Geometry: final body of the model. Coordinates: model frame, mm. Round coordinates to 2 decimals unless told otherwise and drop trailing zeros. Order: outer loops, then holes, each group sorted by start corner. A loop starts at its lowest first (then second) coordinate and runs counter-clockwise, first axis right, second up. Notation, with made-up numbers: M 44,-39 L 73,-39 A17 ccw 73,-17 Z; hole C 36,81 d6. An arc over 180 degrees is marked long. Return JSON: item names as keys, results as strings. Group by question number.
Q1. Cut plane A-A on z = 1.7. Output: boundary loops of the cut face in (x, y).
Q2. Ray query, probe 1 along X at (y, z) = (20, 2.35); probe 2 along Y at (x, z) = (-14.6, 1.35); probe 3 along X at (y, z) = (32, 1.55). Return the intervals inside material, ascending.
Q3. Cut plane B-B on x = -410.5. Output: boundary loops of the cut face in (y, z) (3 decimals).
Q4. Contact query for flat-ended pins moving along their axis: pin 1 (1 mm diameter, centred on x = -445.5, z = 1, fed in from -Y); pin 2 (2 mm diameter, centred on x = -304, y = 116, fed in from -Z). Output: stop coordinate, or through.
Q5. Cut plane C-C on y = 30.5. Output: boundary loops of the cut face in (x, z) (3 decimals), and give its area (3 significant figures).
```python
from build123d import *

# Parameters (mm, degrees)
SKETCH1_R           = 3.05
BOSS_EXTRUDE1_DEPTH = 3.175


with BuildPart() as part:
    # Sketch1 → Boss-Extrude1 (new body)
    with BuildSketch(Plane.XY):
        with BuildLine():
            Line((-466, 88.2), (-466, 131.8))
            Line((-466, 131.8), (0, 131.8))
            Line((0, 131.8), (0, 0))
            Line((0, 0), (-389.2, 0))
            Line((-389.2, 0), (-389.2, 37))
            ThreePointArc((-389.2, 37), (-390.371572875, 39.828427125), (-393.2, 41))
            Line((-393.2, 41), (-429.2, 41))
            Line((-429.2, 41), (-429.2, 80.2))
            ThreePointArc((-429.2, 80.2), (-430.371572875, 83.028427125), (-433.2, 84.2))
            Line((-433.2, 84.2), (-462, 84.2))
            ThreePointArc((-462, 84.2), (-464.828427125, 85.371572875), (-466, 88.2))
        make_face()
        with Locations(Location((-14.6, 20, 0), (0, 0, 180))):
            Circle(SKETCH1_R, mode=Mode.SUBTRACT)
        with Locations(Location((-134.6, 20, 0), (0, 0, 180))):
            Circle(SKETCH1_R, mode=Mode.SUBTRACT)
        with Locations(Location((-254.6, 20, 0), (0, 0, 180))):
            Circle(SKETCH1_R, mode=Mode.SUBTRACT)
        with Locations(Location((-374.6, 20, 0), (0, 0, 180))):
            Circle(SKETCH1_R, mode=Mode.SUBTRACT)
    extrude(amount=BOSS_EXTRUDE1_DEPTH)


solid = part.part
```
Result sheet:
{
 "1": {"outline": "M -466,88.2 A4 ccw -462,84.2 L -433.2,84.2 A4 cw -429.2,80.2 L -429.2,41 L -393.2,41 A4 cw -389.2,37 L -389.2,0 L 0,0 L 0,131.8 L -466,131.8 Z; hole C -374.6,20 d6.1; hole C -254.6,20 d6.1; hole C -134.6,20 d6.1; hole C -14.6,20 d6.1"},
 "2": {"probe 1": "x = -389.2 to -377.65, -371.55 to -257.65, -251.55 to -137.65, -131.55 to -17.65, -11.55 to 0", "probe 2": "y = 0 to 16.95, 23.05 to 131.8", "probe 3": "x = -389.2 to 0"},
 "3": {"outline": "M 41,0 L 131.8,0 L 131.8,3.175 L 41,3.175 Z"},
 "4": {"pin 1": "stops at y = 84.2", "pin 2": "stops at z = 0"},
 "5": {"outline": "M -389.2,0 L 0,0 L 0,3.175 L -389.2,3.175 Z", "area": "1,240 mm²"}
}
